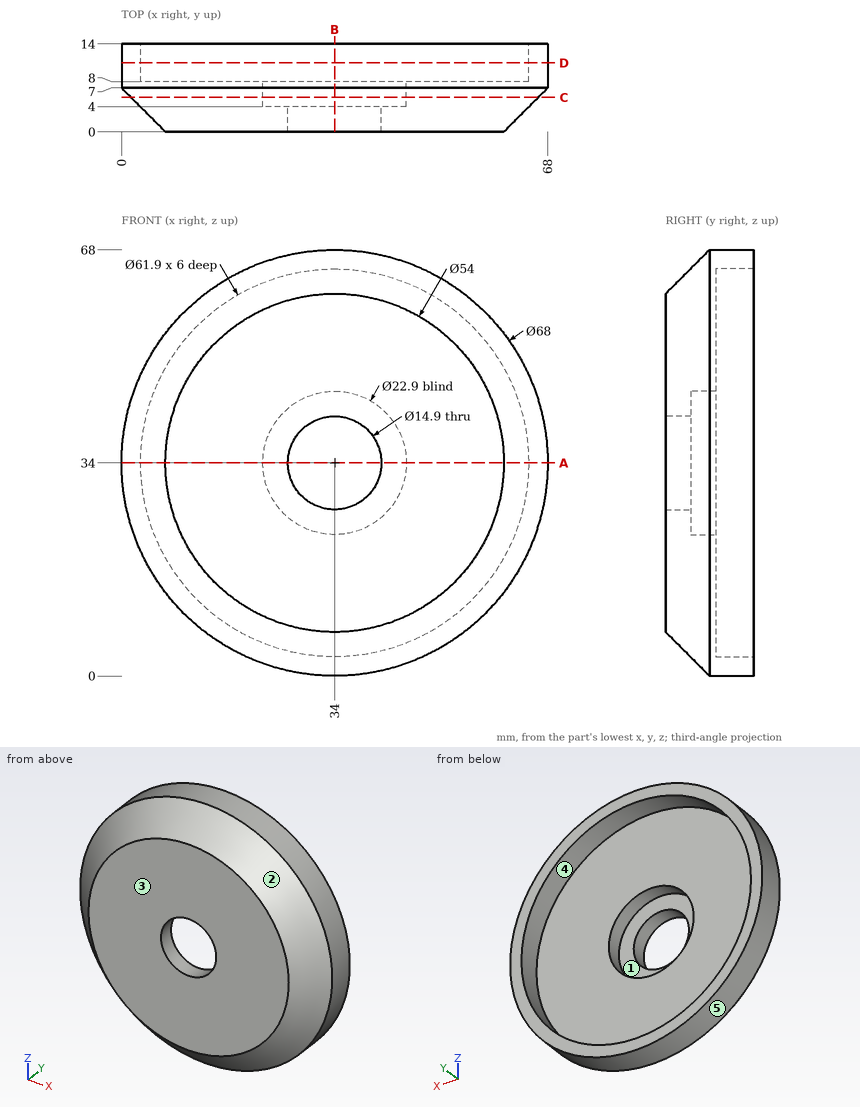
Answer from the drawing. Dimensions are ordinates in mm from the lowest x, y and z of the part. A direction names the side the tool comes from. Round coordinates to 2 decimals unless told otherwise and drop trailing zeros. Loops run counter-clockwise (first coordinate to the right, second up) from the corner with the lowest first, then second, coordinate; pieces in that order, holes last. Notation, with made-up numbers: (-7.75, 46) - (44.25, 46) arc R28 cw to (44.25, 70) - close; hole circle Ø8 at (-20, 68). An arc over 180 degrees is marked (long way). Return JSON: item names as keys, results as strings. Group by question number.
1. Each of these flat-tipped pins is pushed along its axis until it touches: P1, Ø2, axis at x = 28.5, z = 48, coming from the +Y side; P2, Ø4, axis at x = 41, y = 9, coming from the +Z side; P3, Ø13.5, axis at x = 34, z = 34, coming from the +Y side; P4, Ø5, axis at y = 3, z = 54.5, coming from the -X side. Where does it stop, or does it pass through?
2. The part is cut by section B-B on x = 34. Determine the outline of the cut face in (y, z).
3. Which of the six approach directions +Z, -Z, +X, -X, +Y, -Y give full straight-line access (tool end or side, diameter ignored) to the marked faces 1 and 2?
4. The part is cut by section C-C on y = 5.5. Determine the outline of the cut face in (x, z).
5. The mould has two halves that part along X. Classify the marked faces 3, 4 and 5: pulls with the +X half, pulls with the -X half, needs draft (parallel to the pull), parting line crosses it, or undercut.
6. Consider probe 1 along X at (y, z) = (11.4, 34); probe 2 along Y at (x, z) = (10.5, 44); probe 3 along Z at (x, y) = (62, 10). Determine where each line is inside the solid, lowest interval first.
7. The part is cut by section A-A on z = 34. Determine the outline of the cut face in (x, y).
8. The part is cut by section D-D on y = 11. Determine the outline of the cut face in (x, z).
Resolved:
{
 "1": {"P1": "stops at y = 8", "P2": "stops at z = 67.63", "P3": "passes through", "P4": "stops at x = 8.23"},
 "2": {"outline": "(0, 7) - (7, 0) - (14, 0) - (14, 3.05) - (8, 3.05) - (8, 22.55) - (4, 22.55) - (4, 26.55) - (0, 26.55) - close; (0, 41.45) - (4, 41.45) - (4, 45.45) - (8, 45.45) - (8, 64.95) - (14, 64.95) - (14, 68) - (7, 68) - (0, 61) - close"},
 "3": {"face 1": "+Y", "face 2": "-Y"},
 "4": {"outline": "circle Ø65 at (34, 34); hole circle Ø22.9 at (34, 34)"},
 "5": {"face 3": "needs draft", "face 4": "undercut", "face 5": "parting line crosses it"},
 "6": {"probe 1": "x = 0 to 3.05, 64.95 to 68", "probe 2": "y = 0 to 8", "probe 3": "z = 14.71 to 20.81, 47.19 to 53.29"},
 "7": {"outline": "(0, 7) - (7, 0) - (26.55, 0) - (26.55, 4) - (22.55, 4) - (22.55, 8) - (3.05, 8) - (3.05, 14) - (0, 14) - close; (41.45, 0) - (61, 0) - (68, 7) - (68, 14) - (64.95, 14) - (64.95, 8) - (45.45, 8) - (45.45, 4) - (41.45, 4) - close"},
 "8": {"outline": "circle Ø68 at (34, 34); hole circle Ø61.9 at (34, 34)"}
}
